Geometry: final body of the model. Coordinates: model frame, mm. A direction names the side the tool comes from. Round coordinates to 2 decimals unless told otherwise and drop trailing zeros. Order: outer loops, then holes, each group sorted by start corner. A loop starts at its lowest first (then second) coordinate and runs counter-clockwise, first axis right, second up. Notation, with made-up numbers: (0.5, 71.25) -> (10.5, 71.25) arc R23 ccw to (10.5, 100.25) -> close; hole circle Ø11 at (17, 56.5). An arc over 180 degrees is marked (long way). Put each result on its own line as item: value.
```python
from build123d import *

# Parameters (mm, degrees)
F0_W     = 125
F0_H     = 75
F1_DEPTH = 15
F3_DEPTH = 15
F3_TAPER = -3


with BuildPart() as f1:
    # F0 (on Top) → F1 (new body)
    with BuildSketch(Plane.XY):
        Rectangle(F0_W, F0_H)
    extrude(amount=F1_DEPTH)

    # F2 (on face) → F3 (join)
    with BuildSketch(Plane.XZ.offset(37.5)):
        with BuildLine():
            Line((7.5, 50), (25, 50))
            ThreePointArc((25, 50), (0, 75), (-25, 50))
            Line((-25, 50), (-7.5, 50))
            ThreePointArc((-7.5, 50), (0, 57.5), (7.5, 50))
        make_face()
        with BuildLine():
            ThreePointArc((-25, 50), (0, 25), (25, 50))
            Line((25, 50), (7.5, 50))
            ThreePointArc((7.5, 50), (0, 42.5), (-7.5, 50))
            Line((-7.5, 50), (-25, 50))
        make_face()
        with BuildLine():
            Line((25, 15), (25, 50))
            ThreePointArc((25, 50), (0, 25), (-25, 50))
            Line((-25, 50), (-25, 15))
            Line((-25, 15), (25, 15))
        make_face()
    extrude(amount=-F3_DEPTH, taper=F3_TAPER)


solid = f1.part
```
1. Cut plane A-A on x = 0. Return loops of the section in (y, z).
Ans:
outline: (-37.5, 0) -> (37.5, 0) -> (37.5, 15) -> (-22.5, 15) -> (-22.5, 43.29) -> (-37.5, 42.5) -> close; (-37.5, 57.5) -> (-22.5, 56.71) -> (-22.5, 75.79) -> (-37.5, 75) -> close
2. Draft query along X for faces 1 (the face through (3.28, -29.9, 56.3)), 2 (the face through (-1, 37.5, 7)), 3 (the face through (0.558, -29.895, 75.392)), 4 (the face through (62.5, -1, 7)). Return one class per face: +X half, -X half, draft (parallel to the pull), parting line (faces both ways), or undercut.
Ans:
face 1: undercut
face 2: draft
face 3: parting line
face 4: +X half
3. Material intervals for probe 1 along Y at (x, z) = (11.5, 29.5); probe 2 along Z at (x, y) = (40.5, -29.5); probe 3 along X at (y, z) = (-25, 51.5), sorted ascending.
Ans:
probe 1: -37.5 to -22.5
probe 2: 0 to 15
probe 3: -25.61 to -6.68, 6.68 to 25.61
4. Cut plane B-B on x = -47.5. Return loops of the section in (y, z).
Ans:
outline: (-37.5, 0) -> (37.5, 0) -> (37.5, 15) -> (-37.5, 15) -> close
5. Set-up query: faces 5 (the face through (0, -22.5, 38)), 6 (the face through (-62.5, -1, 7)). Return all of +Z, -Z, +X, -X, +Y, -Y with unobstructed straight access to the full face (end or side cutting, diameter ignored); none if empty.
Ans:
face 5: +Z, +X, -X, +Y
face 6: +Z, -Z, -X, +Y, -Y
6. Contact query for a flat-ended pin moving along its axis: P1, Ø4, axis at x = 27, z = 49.5, coming from the +Y side. Output: stop coordinate, or through.
Ans:
P1: y = -22.5
